Here's how the part is built. I have some questions about the finished solid (model axes, mm). Coordinates: 2 decimals unless noted, no trailing zeros. Write each loop counter-clockwise with the first axis right and the second up, starting at its lowest first coordinate (ties: lowest second). Pieces come first, ordered by that corner, then holes.
Item 1: If we section it at C-C (x = -20): Please give me the cut outline in (y, z).
Item 2: I'm going to push a flat-ended pin straight in: pin 1 Ø4.5 at (x, y) = (20, 0) entering from -Z. Where does the tip first touch, or does it pass through?
Item 3: If we section it at A-A (x = 0): Please give me the cut outline in (y, z).
Item 4: If we section it at B-B (y = 4): Please give me the cut outline in (x, z).
Item 5: If we section it at D-D (z = 1.8): Please give me the cut outline in (x, y), then the cut area to 3 significant figures.
Item 6: If I drill on line 1 (Y direction, x = 20, z = 3.05); line 2 (X direction, y = -0.5, z = 0.95); line 3 (X direction, y = -3.5, z = 3.05), over which ranges is the centre line in solid material (lowest first)?
from build123d import *

# Parameters (mm, degrees)
F0_W     = 50
F0_H     = 60
F0_R     = 2.5
F0_W_2   = 27
F0_H_2   = 19
F1_DEPTH = 4
F2_R     = 2


with BuildPart() as f1:
    # F0 (on Top) → F1 (new body)
    with BuildSketch(Plane.XY):
        Rectangle(F0_W, F0_H)
        with Locations((0, -20)):
            Circle(F0_R, mode=Mode.SUBTRACT)
        with Locations((-20, 0)):
            Circle(F0_R, mode=Mode.SUBTRACT)
        Rectangle(F0_W_2, F0_H_2, mode=Mode.SUBTRACT)
        with Locations((20, 0)):
            Circle(F0_R, mode=Mode.SUBTRACT)
        with Locations((0, 20)):
            Circle(F0_R, mode=Mode.SUBTRACT)
    extrude(amount=F1_DEPTH)

    # F2
    f2_edges = [f1.edges().sort_by_distance(p)[0] for p in [
        (25, 30, 2),
        (25, -30, 2),
        (-25, 30, 2),
        (-25, -30, 2),
    ]]
    fillet(f2_edges, radius=F2_R)


solid = f1.part
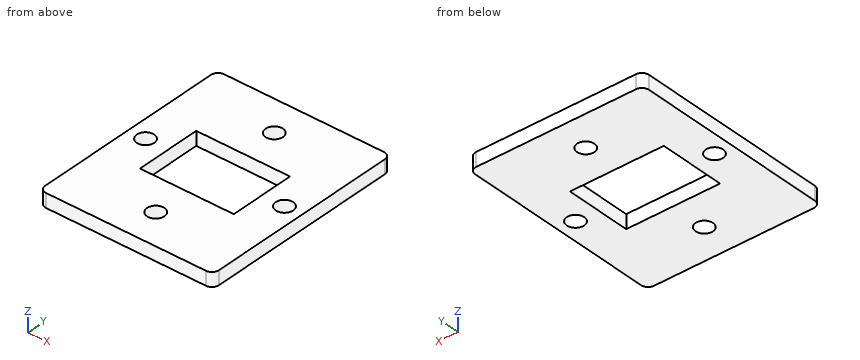
Answer list:
1. outline: (-30, 0) - (-2.5, 0) - (-2.5, 4) - (-30, 4) - close; (2.5, 0) - (30, 0) - (30, 4) - (2.5, 4) - close
2. pin 1: passes through
3. outline: (-30, 0) - (-22.5, 0) - (-22.5, 4) - (-30, 4) - close; (-17.5, 0) - (-9.5, 0) - (-9.5, 4) - (-17.5, 4) - close; (9.5, 0) - (17.5, 0) - (17.5, 4) - (9.5, 4) - close; (22.5, 0) - (30, 0) - (30, 4) - (22.5, 4) - close
4. outline: (-25, 0) - (-13.5, 0) - (-13.5, 4) - (-25, 4) - close; (13.5, 0) - (25, 0) - (25, 4) - (13.5, 4) - close
5. outline: (-25, -28) arc R2 ccw to (-23, -30) - (23, -30) arc R2 ccw to (25, -28) - (25, 28) arc R2 ccw to (23, 30) - (-23, 30) arc R2 ccw to (-25, 28) - close; hole circle Ø5 at (-20, 0); hole (-13.5, -9.5) - (13.5, -9.5) - (13.5, 9.5) - (-13.5, 9.5) - close; hole circle Ø5 at (0, -20); hole circle Ø5 at (0, 20); hole circle Ø5 at (20, 0)
5. area: 2,410 mm2
6. line 1: y = -30 to -2.5, 2.5 to 30
6. line 2: x = -25 to -22.45, -17.55 to -13.5, 13.5 to 17.55, 22.45 to 25
6. line 3: x = -25 to -13.5, 13.5 to 25
